Part print with two shaded views. Sizes in mm from the minimum x, y, z corner. Round coordinates to 2 decimals unless told otherwise and drop trailing zeros. Loops run counter-clockwise (first coordinate to the right, second up) from the corner with the lowest first, then second, coordinate; pieces in that order, holes last. Notation, with made-up numbers: (88.5, 51.5) - (134.5, 51.5) arc R26 cw to (134.5, 73.5) - close; hole circle Ø10 at (34, -33.75). An arc over 180 degrees is marked (long way). One line per question, with ' | ' between items.
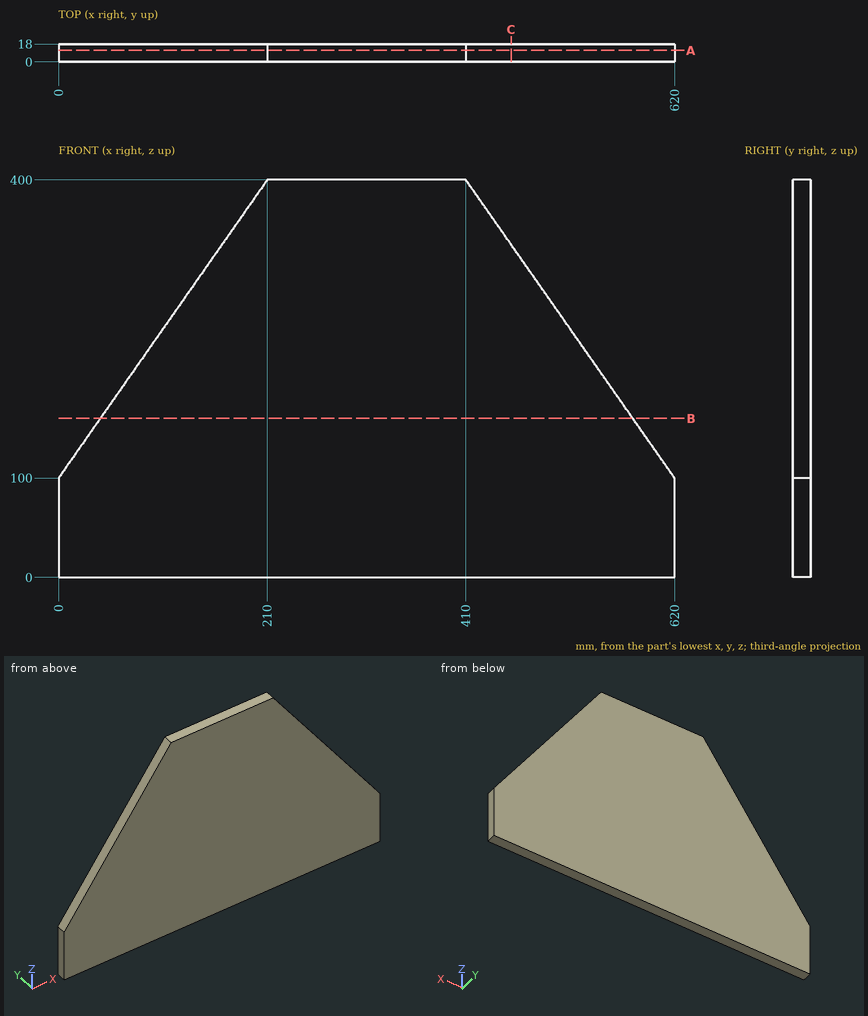
(1) Cut at C-C, the plane x = 455.5. Write the cut outline in (y, z), then the cut area to 3 significant figures.
Results found:
outline: (0, 0) - (18, 0) - (18, 335) - (0, 335) - close | area: 6,030 mm²
(2) Probe L1, parallel to X at y = 15.75, z = 219.5; L2, parallel to X at y = 15, z = 179; L3, parallel to Z at x = 560.5, y = 1.5. List the from-to ranges inside material, lowest first.
Results found:
L1: x = 83.65 to 536.35 | L2: x = 55.3 to 564.7 | L3: z = 0 to 185
(3) Cut at A-A, the plane y = 11.5. Write the cut outline in (x, z).
Results found:
outline: (0, 0) - (620, 0) - (620, 100) - (410, 400) - (210, 400) - (0, 100) - close
(4) Cut at B-B, the plane z = 160. Write the cut outline in (x, y).
Results found:
outline: (42, 0) - (578, 0) - (578, 18) - (42, 18) - close
(5) Drop flat-ended pins along their axis: P1, Ø4, axis at y = 8.5, z = 144, coming from the -X side; P2, Ø5, axis at x = 70, y = 13.5, coming from the +Z side; P3, Ø2, axis at x = 498.5, y = 9, coming from the +Z side. Give the stop position or say it passes through.
Results found:
P1: stops at x = 29.4 | P2: stops at z = 203.57 | P3: stops at z = 275
